```python
from build123d import *

# Parameters (mm, degrees)
SKETCH3_W           = 38
SKETCH3_H           = 34
SKETCH3_W_2         = 26
SKETCH3_H_2         = 22
BOSS_EXTRUDE1_DEPTH = 22
SKETCH4_W           = 24
SKETCH4_H           = 22
BOSS_EXTRUDE2_DEPTH = 1
SKETCH5_R           = 2.7
CUT_EXTRUDE1_DEPTH  = 12
SKETCH7_R           = 5.7
CUT_EXTRUDE3_DEPTH  = 4.2
SKETCH8_R           = 6.2
CUT_EXTRUDE4_DEPTH  = 57.151580565
SKETCH9_R           = 9.2
CUT_EXTRUDE5_DEPTH  = 4.2
SKETCH10_R          = 9.2
CUT_EXTRUDE6_DEPTH  = 4.2
SKETCH15_R          = 1.45
CUT_EXTRUDE7_DEPTH  = 57.151580565
FILLET1_R           = 3
FILLET3_R           = 2.5
FILLET4_R           = 2.2
FILLET5_R           = 2.4


with BuildPart() as part:
    # Sketch3 → Boss-Extrude1 (new body)
    with BuildSketch(Plane(origin=(0, 0, 0), x_dir=(1, 0, 0), z_dir=(0, 1, 0))):
        with Locations((19, -17)):
            Rectangle(SKETCH3_W, SKETCH3_H)
        with Locations((19, -17)):
            Rectangle(SKETCH3_W_2, SKETCH3_H_2, mode=Mode.SUBTRACT)
    extrude(amount=BOSS_EXTRUDE1_DEPTH)

    # Sketch4 → Boss-Extrude2 (add)
    with BuildSketch(Plane.XY.offset(34)):
        with Locations((19, 11)):
            Rectangle(SKETCH4_W, SKETCH4_H)
    extrude(amount=BOSS_EXTRUDE2_DEPTH)

    # Sketch5 → Cut-Extrude1 (cut)
    with BuildSketch(Plane.XY.offset(35)):
        with Locations((19, 11)):
            Circle(SKETCH5_R)
    extrude(amount=-CUT_EXTRUDE1_DEPTH, mode=Mode.SUBTRACT)

    # Sketch7 → Cut-Extrude3 (cut)
    with BuildSketch(Plane(origin=(0, 0, 28), x_dir=(-1, 0, 0), z_dir=(0, 0, -1))):
        with Locations((-19, 11)):
            Circle(SKETCH7_R)
    extrude(amount=-CUT_EXTRUDE3_DEPTH, mode=Mode.SUBTRACT)

    # Sketch8 → Cut-Extrude4 (cut, through all)
    with BuildSketch(Plane(origin=(38, 0, 0), x_dir=(0, 0, -1), z_dir=(1, 0, 0))):
        with Locations((-15, 11)):
            Circle(SKETCH8_R)
    extrude(amount=-CUT_EXTRUDE4_DEPTH, mode=Mode.SUBTRACT)

    # Sketch9 → Cut-Extrude5 (cut)
    with BuildSketch(Plane(origin=(6, 0, 0), x_dir=(0, 0, -1), z_dir=(1, 0, 0))):
        with Locations((-15, 11)):
            Circle(SKETCH9_R)
    extrude(amount=-CUT_EXTRUDE5_DEPTH, mode=Mode.SUBTRACT)

    # Sketch10 → Cut-Extrude6 (cut)
    with BuildSketch(Plane(origin=(38, 0, 0), x_dir=(0, 0, -1), z_dir=(1, 0, 0))):
        with Locations((-15, 11)):
            Circle(SKETCH10_R)
    extrude(amount=-CUT_EXTRUDE6_DEPTH, mode=Mode.SUBTRACT)

    # Sketch15 → Cut-Extrude7 (cut, through all)
    with BuildSketch(Plane(origin=(0, 0, 0), x_dir=(-1, 0, 0), z_dir=(0, -1, 0))):
        with Locations(Location((-4, -30, 0), (0, 0, 90))):
            Circle(SKETCH15_R)
        with Locations(Location((-34, -30, 0), (0, 0, 90))):
            Circle(SKETCH15_R)
        with Locations(Location((-34, -4, 0), (0, 0, 90))):
            Circle(SKETCH15_R)
        with Locations(Location((-4, -4, 0), (0, 0, 90))):
            Circle(SKETCH15_R)
    extrude(amount=-CUT_EXTRUDE7_DEPTH, mode=Mode.SUBTRACT)

    # Fillet1
    # the kernel refuses this fillet: 3 mm, written as the material it takes off along each edge
    with BuildSketch(Plane(origin=(38, -7.5, 0), x_dir=(-1, 0, 0), z_dir=(0, 1, 0)), Plane(origin=(38, -7.5, 34), x_dir=(0, 0, -1), z_dir=(0, 1, 0))) as fillet1_piece_1:
        with BuildLine():
            CenterArc((FILLET1_R, FILLET1_R), FILLET1_R, 180, 90)
            Line((0, FILLET1_R), (-FILLET1_R * 0.02, FILLET1_R))
            Line((-FILLET1_R * 0.02, FILLET1_R), (-FILLET1_R * 0.02, -FILLET1_R * 0.02))
            Line((-FILLET1_R * 0.02, -FILLET1_R * 0.02), (FILLET1_R, -FILLET1_R * 0.02))
            Line((FILLET1_R, -FILLET1_R * 0.02), (FILLET1_R, 0))
        make_face()
    extrude(amount=37, mode=Mode.SUBTRACT)
    with BuildSketch(Plane(origin=(7, -5.590169944, 35), x_dir=(0, 0, -1), z_dir=(0, 1, 0)), Plane(origin=(31, 27.590169944, 35), x_dir=(0, 0, -1), z_dir=(0, -1, 0))) as fillet1_piece_2:
        with BuildLine():
            CenterArc((3, -2.236067977), FILLET1_R, 131.810314896, 48.189685104)
            Line((0, -2.236067977), (-0.06, -2.236067977))
            Line((-0.06, -2.236067977), (-0.06, 0))
            Line((-0.06, 0), (0, 0.06))
            ThreePointArc((0, 0.06), (0.5, 0.06), (0.96, 0.04472136))
            Line((0.96, 0.04472136), (1, 0))
        make_face()
    extrude(amount=33.180339887, mode=Mode.SUBTRACT)
    with BuildSketch(Plane(origin=(0, -7.5, 34), x_dir=(0, 0, -1), z_dir=(0, 1, 0)), Plane(origin=(0, -7.5, 0), x_dir=(1, 0, 0), z_dir=(0, 1, 0))) as fillet1_piece_3:
        with BuildLine():
            CenterArc((FILLET1_R, -FILLET1_R), FILLET1_R, 90, 90)
            Line((0, -FILLET1_R), (-FILLET1_R * 0.02, -FILLET1_R))
            Line((-FILLET1_R * 0.02, -FILLET1_R), (-FILLET1_R * 0.02, FILLET1_R * 0.02))
            Line((-FILLET1_R * 0.02, FILLET1_R * 0.02), (FILLET1_R, FILLET1_R * 0.02))
            Line((FILLET1_R, FILLET1_R * 0.02), (FILLET1_R, 0))
        make_face()
    extrude(amount=37, mode=Mode.SUBTRACT)

    # Fillet3
    fillet3_edges = [part.edges().sort_by_distance(p)[0] for p in [
        (6, 11, 28),
        (32, 11, 6),
    ]]
    fillet(fillet3_edges, radius=FILLET3_R)

    # Fillet4
    fillet4_edges = [part.edges().sort_by_distance(p)[0] for p in [
        (32, 11, 28),
    ]]
    fillet(fillet4_edges, radius=FILLET4_R)

    # Fillet5
    # the kernel refuses this fillet: 2.4 mm, written as the material it adds along each edge
    with BuildSketch(Plane(origin=(6, 6.907878403, 6), x_dir=(0, 0, 1), z_dir=(0, 1, 0))) as fillet5_piece_1_section:
        with BuildLine():
            CenterArc((FILLET5_R, FILLET5_R), FILLET5_R, 180, 90)
            Line((0, FILLET5_R), (0, 0))
            Line((0, 0), (FILLET5_R, 0))
        make_face()
    fillet5_piece_1 = extrude(amount=15.092121597, mode=Mode.PRIVATE)
    fillet5_piece_1 = fillet5_piece_1 - Plane(origin=(6.778295216, 11, 15), x_dir=(0, 0, -1), z_dir=(1, 0, 0)) * Cylinder(9.2, 40, mode=Mode.PRIVATE)
    add(fillet5_piece_1)
    with BuildSketch(Plane(origin=(6, 0, 6), x_dir=(0, 0, 1), z_dir=(0, 1, 0))) as fillet5_piece_2_section:
        with BuildLine():
            CenterArc((FILLET5_R, FILLET5_R), FILLET5_R, 180, 90)
            Line((0, FILLET5_R), (0, 0))
            Line((0, 0), (FILLET5_R, 0))
        make_face()
    fillet5_piece_2 = extrude(amount=15.092121597, mode=Mode.PRIVATE)
    fillet5_piece_2 = fillet5_piece_2 - Plane(origin=(6.572967992, 11, 15), x_dir=(0, 0, -1), z_dir=(1, 0, 0)) * Cylinder(9.2, 40, mode=Mode.PRIVATE)
    add(fillet5_piece_2)


solid = part.part
```
Work out the finished part from the listing and answer in its coordinate system (mm). A direction names the side the tool comes from. Coordinates: 2 decimals unless noted, no trailing zeros. Write each loop counter-clockwise with the first axis right and the second up, starting at its lowest first coordinate (ties: lowest second). Pieces come first, ordered by that corner, then holes.
Q1. Which of the six approach directions +Z, -Z, +X, -X, +Y, -Y give full straight-line access (tool end or side, diameter ignored) to faces 1 (the face through (1.8, 5, 17.2)), 2 (the face through (20.452, 13.277, 33.62)), 3 (the face through (31.34, 11.15, 27.37)), 4 (the face through (35.929, 13.763, 6.225)), 5 (the face through (0.9, 10.85, 0.86))?
Q2. A cutting plane is placed at A-A, the plane z = 30. Give the vertices of the cut face in (x, y), then the cut area to 3 significant figures.
Q3. A cutting plane is placed at D-D, the plane y = 11. State how many separate pieces and enclosed holes the cut face has, then the cut area to 3 significant figures.
Q4. This flat-tipped pin is pushed along its axis until it touches: pin 1 Ø1 at (y, z) = (14, 8) entering from +X. Where does it stop, or does it pass through?
Q5. A cutting plane is placed at B-B, the plane x = 19. Give the vertices of the cut face in (y, z), then the cut area to 3 significant figures.
Q6. A cutting plane is placed at C-C, the plane z = 15. Give the vertices of the cut face in (x, y), then the cut area to 3 significant figures.
Q7. Determine the mould class of faces 6 (the face through (0.86, 10.85, 33.1)), 7 (the face through (19, 11, 0)), 8 (the face through (6.752, 11.154, 27.287)) for opening direction X: released by +X, released by -X, zero draft, split by the parting line, or undercut.
Q8. Find the intervals of material crossed by line 1 (X direction, y = 13, z = 4); line 2 (X direction, y = 14, z = 23); line 3 (Z direction, x = 27, y = 17.25), in increasing order.
Findings below:
1. face 1: none
1. face 2: +Z
1. face 3: +Y, -Y
1. face 4: +X
1. face 5: -Z, -X, +Y, -Y
2. outline: (0, 0) - (2.55, 0) - (2.55, 22) - (0, 22) - close; (5.45, 0) - (32.55, 0) - (32.55, 22) - (5.45, 22) - close; (35.45, 0) - (38, 0) - (38, 22) - (35.45, 22) - close; hole circle Ø11.4 at (19, 11)
2. area: 606 mm2
3. separate pieces: 3
3. enclosed holes: 4
3. area: 450 mm2
4. pin 1: stops at x = 33.8
5. outline: (0, 0) - (22, 0) - (22, 6) - (0, 6) - close; (0, 28) - (5.3, 28) - (5.3, 32.2) - (8.3, 32.2) - (8.3, 35) - (0, 35) - close; (13.7, 32.2) - (16.7, 32.2) - (16.7, 28) - (22, 28) - (22, 35) - (13.7, 35) - close
5. area: 223 mm2
6. outline: (0, 0) - (6, 0) - (6, 1.8) - (1.8, 1.8) - (1.8, 4.8) - (0, 4.8) - close; (0, 17.2) - (1.8, 17.2) - (1.8, 20.2) - (6, 20.2) - (6, 22) - (0, 22) - close; (32, 0) - (38, 0) - (38, 1.8) - (33.8, 1.8) - (33.8, 4.8) - (32, 4.8) - close; (32, 17.2) - (33.8, 17.2) - (33.8, 20.2) - (38, 20.2) - (38, 22) - (32, 22) - close
6. area: 64.8 mm2
7. face 6: released by -X
7. face 7: zero draft
7. face 8: undercut
8. line 1: x = 0 to 2.55, 5.45 to 32.55, 35.45 to 38
8. line 2: x = 0 to 1.8, 32 to 33.8
8. line 3: z = 0 to 6, 28 to 35
